Geometry check sheet. Reference: the model listing, model coordinates, mm. A direction names the side the tool comes from. Round coordinates to 2 decimals unless told otherwise and drop trailing zeros. Write each loop counter-clockwise with the first axis right and the second up, starting at its lowest first coordinate (ties: lowest second). Pieces come first, ordered by that corner, then holes. Notation, with made-up numbers: (31, 58.5) -> (77, 58.5) arc R18 ccw to (77, 64.5) -> close; hole circle Ø2 at (-36.75, 43.5). An arc over 180 degrees is marked (long way). Return JSON: item names as keys, results as strings. Group by question number.
from build123d import *

# Parameters (mm, degrees)
SALIENTE_EXTRUIR1_DEPTH      = 30
SALIENTE_EXTRUIR1_DEPTH_BACK = 30
CROQUIS3_R                   = 1.75
CORTAR_EXTRUIR1_DEPTH        = 4.242641
CROQUIS4_R                   = 3
CORTAR_EXTRUIR2_DEPTH        = 2
CROQUIS5_R                   = 10
CROQUIS5_R_2                 = 1.75
CORTAR_EXTRUIR3_DEPTH        = 6
CROQUIS5_4_R                 = 12.5
CROQUIS5_4_R_2               = 10
CORTAR_EXTRUIR4_DEPTH        = 4.4
REDONDEO1_R                  = 10
REDONDEO2_R                  = 3
REDONDEO3_R                  = 10
CROQUIS6_R                   = 2.06
CORTAR_EXTRUIR5_DEPTH        = 4.2


with BuildPart() as part:
    # Croquis2 → Saliente-Extruir1 (new body, two sides)
    with BuildSketch(Plane(origin=(0, 0, 0), x_dir=(0, 0, -1), z_dir=(1, 0, 0))) as saliente_extruir1_sk:
        Polygon((0, 0), (-28, 0), (-28, 6), (0, 6), (14.960512242, 20.960512242), (17.960512242, 17.960512242), align=None)
    extrude(amount=SALIENTE_EXTRUIR1_DEPTH)
    extrude(saliente_extruir1_sk.sketch, amount=-SALIENTE_EXTRUIR1_DEPTH_BACK)

    # Croquis3 → Cortar-Extruir1 (cut)
    with BuildSketch(Plane(origin=(0, 0, 0), x_dir=(-1, 0, 0), z_dir=(0, -0.707106781, -0.707106781))):
        with Locations((-25, 12.7)):
            Circle(CROQUIS3_R)
        with Locations((25, 12.7)):
            Circle(CROQUIS3_R)
    extrude(amount=-CORTAR_EXTRUIR1_DEPTH, mode=Mode.SUBTRACT)

    # Croquis4 → Cortar-Extruir2 (cut)
    with BuildSketch(Plane(origin=(0, 3, 3), x_dir=(1, 0, 0), z_dir=(0, 0.707106781, 0.707106781))):
        with Locations((-25, 12.7)):
            Circle(CROQUIS4_R)
        with Locations((25, 12.7)):
            Circle(CROQUIS4_R)
    extrude(amount=-CORTAR_EXTRUIR2_DEPTH, mode=Mode.SUBTRACT)

    # Croquis5 → Cortar-Extruir3 (cut)
    with BuildSketch(Plane(origin=(0, 0, 0), x_dir=(-1, 0, 0), z_dir=(0, -1, 0))):
        with Locations((0, -14)):
            Circle(CROQUIS5_R)
        with Locations((14.5, -23)):
            Circle(CROQUIS5_R_2)
        with Locations((-14.5, -23)):
            Circle(CROQUIS5_R_2)
        with BuildLine():
            ThreePointArc((-19.082136833, -25.001005257), (-17.238153914, -27.1836005), (-14.5, -28))
            Line((-14.5, -28), (-30, -28))
            Line((-30, -28), (-30, 0))
            Line((-30, 0), (-19.082136833, -25.001005257))
        make_face()
        with BuildLine():
            Line((30, 0), (19.082136833, -25.001005257))
            ThreePointArc((19.082136833, -25.001005257), (17.238153914, -27.1836005), (14.5, -28))
            Line((14.5, -28), (30, -28))
            Line((30, -28), (30, 0))
        make_face()
    extrude(amount=-CORTAR_EXTRUIR3_DEPTH, mode=Mode.SUBTRACT)

    # Croquis5<4> → Cortar-Extruir4 (cut)
    with BuildSketch(Plane(origin=(0, 0, 0), x_dir=(-1, 0, 0), z_dir=(0, -1, 0))):
        with Locations((0, -14)):
            Circle(CROQUIS5_4_R)
        with Locations((0, -14)):
            Circle(CROQUIS5_4_R_2, mode=Mode.SUBTRACT)
    extrude(amount=-CORTAR_EXTRUIR4_DEPTH, mode=Mode.SUBTRACT)

    # Redondeo1
    redondeo1_edges = [part.edges().sort_by_distance(p)[0] for p in [
        (0, 6, 0),
    ]]
    fillet(redondeo1_edges, radius=REDONDEO1_R)

    # Redondeo2
    redondeo2_edges = [part.edges().sort_by_distance(p)[0] for p in [
        (0, 0, 0),
    ]]
    fillet(redondeo2_edges, radius=REDONDEO2_R)

    # Redondeo3
    redondeo3_edges = [part.edges().sort_by_distance(p)[0] for p in [
        (-30, 3.583831813, 0),
        (30, 3.583831813, 0),
    ]]
    fillet(redondeo3_edges, radius=REDONDEO3_R)

    # Croquis6 → Cortar-Extruir5 (cut)
    with BuildSketch(Plane(origin=(0, 6, 0), x_dir=(1, 0, 0), z_dir=(0, 1, 0))):
        with Locations((-14.5, -23)):
            Circle(CROQUIS6_R)
        with Locations((14.5, -23)):
            Circle(CROQUIS6_R)
    extrude(amount=-CORTAR_EXTRUIR5_DEPTH, mode=Mode.SUBTRACT)


solid = part.part
1) Go/stop test with flat-tipped pins: P1, Ø1.5, axis at x = 5, y = 9, coming from the +Z side; P2, Ø1.5, axis at x = -19, z = 22, coming from the +Y side; P3, Ø3, axis at x = 14.5, z = 23, coming from the +Y side; P4, Ø5, axis at x = -13.5, y = 14.5, coming from the +Z side. Record where each tip stops, or that it passes through.
2) Sectioned sample at B-B on x = -25.5. Enter the section's corners in (y, z), and give its area (3 significant figures).
3) Sectioned sample at A-A on z = 14. Enter the section's corners in (x, y).
4) Mould release check, pull along Z, two halves, no side actions. Record for faces 1 (the face through (30, 12, -9)), 2 (the face through (12.98, 3.93, 21.61)), 3 (the face through (-17.272, 2.958, 27.161)): +Z half, -Z half, draft (parallel to the pull), parting line (faces both ways), or undercut.
5) Sectioned sample at C-C on z = 23. Enter the section's corners in (x, y), and give its area (3 significant figures).
6) Tool access check on faces 4 (the face through (0.4, 6, 24.2)), 5 (the face through (-24.19, 3.08, 13.3)), 6 (the face through (-25.04, 9.18, -6.01)). Record the directions out of +Z, -Z, +X, -X, +Y, -Y that give a thin tool (end or side, any length) a straight path to the whole face; none if there is none.
7) Material ranges on probe 1 along X at (y, z) = (0.7, 23); probe 2 along X at (y, z) = (4.2, 23); probe 3 along X at (y, z) = (13, -8.5), recorded low to high. Write a range as [from, to].
8) Sectioned sample at D-D on y = 15.75. Enter the section's corners in (x, z), and give its area (3 significant figures).
Evaluation:
{
 "1": {"P1": "stops at z = -2.18", "P2": "stops at y = 6", "P3": "passes through", "P4": "stops at z = -6"},
 "2": {"outline": "(0, 1.24) arc R3 ccw to (0.88, -0.88) -> (7.79, -7.79) -> (9.38, -6.21) -> (8.47, -5.3) -> (9.89, -3.89) -> (8.93, -2.93) arc R10 cw to (6, 4.14) -> (6, 10.3) -> (0, 10.3) -> close; (10.17, -10.17) -> (17.96, -17.96) -> (20.96, -14.96) -> (14.07, -8.07) -> (12.66, -9.49) -> (11.75, -8.58) -> close", "area": "143 mm2"},
 "3": {"outline": "(-23.89, 0) -> (-12.5, 0) -> (-12.5, 4.4) -> (-10, 4.4) -> (-10, 6) -> (-23.89, 6) -> close; (10, 4.4) -> (12.5, 4.4) -> (12.5, 0) -> (23.89, 0) -> (23.89, 6) -> (10, 6) -> close"},
 "4": {"face 1": "draft", "face 2": "undercut", "face 3": "+Z half"},
 "5": {"outline": "(-19.96, 0) -> (-16.25, 0) -> (-16.25, 1.8) -> (-16.56, 1.8) -> (-16.56, 6) -> (-19.96, 6) -> close; (-12.75, 0) -> (-8.67, 0) -> (-8.67, 4.4) -> (-4.36, 4.4) -> (-4.36, 6) -> (-12.44, 6) -> (-12.44, 1.8) -> (-12.75, 1.8) -> close; (4.36, 4.4) -> (8.67, 4.4) -> (8.67, 0) -> (12.75, 0) -> (12.75, 1.8) -> (12.44, 1.8) -> (12.44, 6) -> (4.36, 6) -> close; (16.25, 0) -> (19.96, 0) -> (19.96, 6) -> (16.56, 6) -> (16.56, 1.8) -> (16.25, 1.8) -> close", "area": "102 mm2"},
 "6": {"face 4": "+Z, +X, -X, +Y", "face 5": "+Z, -X, +Y, -Y", "face 6": "none"},
 "7": {"probe 1": "x = [-19.96, -16.25], [-12.75, -8.67], [8.67, 12.75], [16.25, 19.96]", "probe 2": "x = [-19.96, -16.56], [-12.44, -8.67], [8.67, 12.44], [16.56, 19.96]", "probe 3": "x = [-30, -26.65], [-23.35, 23.35], [26.65, 30]"},
 "8": {"outline": "(-30, -15.75) -> (30, -15.75) -> (30, -9.75) -> (-30, -9.75) -> close", "area": "360 mm2"}
}
